Input: part model. Units: mm. Frame: model coordinates. A direction names the side the tool comes from. Coordinates: 2 decimals unless noted, no trailing zeros. Write each loop counter-clockwise with the first axis right and the second up, starting at its lowest first coordinate (ties: lowest second). Pieces come first, ordered by that corner, then holes. Notation, with made-up numbers: M 61,-16 L 99,-16 A32 cw 99,22 Z; hole C 65,27.25 d2. An arc over 180 degrees is marked long. Use CSV: the item, a comma, the result in double quotes.
```python
from build123d import *

# Parameters (mm, degrees)
SKETCH_1_W = 1.2
SKETCH_1_H = 5


with BuildPart() as part:
    # 草图1 → 旋转1 (revolve)
    with BuildSketch(Plane(origin=(0, 0, 0), x_dir=(1, 0, 0), z_dir=(0, 1, 0)), mode=Mode.PRIVATE) as revolve_1_sk:
        Polygon((0, 8.7), (0, 6), (1.45, 6), (2.95, 6), (2.95, 8.7), align=None)
        Polygon((0, 6), (0, 0), (1.2, 0), (1.45, 0), (1.45, 6), align=None)
        with Locations((0.6, -2.5)):
            Rectangle(SKETCH_1_W, SKETCH_1_H)
    revolve(revolve_1_sk.sketch.rotate(Axis((0, 0, -34.43030142), (0, 0, 1)), 180), axis=Axis((0, 0, -34.43030142), (0, 0, 1)))


solid = part.part
```
1. Section C-C (z = -5.75). Return loops of the section in (x, y).
Resolved:
outline,"C 0,0 d2.9"
2. Section D-D (y = 1.7). Return loops of the section in (x, z).
Resolved:
outline,"M -2.41,-8.7 L 2.41,-8.7 L 2.41,-6 L -2.41,-6 Z"
3. Section A-A (x = 0). Return loops of the section in (y, z).
Resolved:
outline,"M -2.95,-8.7 L 2.95,-8.7 L 2.95,-6 L 1.45,-6 L 1.45,0 L 1.2,0 L 1.2,5 L -1.2,5 L -1.2,0 L -1.45,0 L -1.45,-6 L -2.95,-6 Z"
4. Contact query for flat-ended pins moving along their axis: pin 1 Ø3 at (y, z) = (1, -2.5) entering from +X; pin 2 Ø3 at (x, z) = (-0.5, 2.5) entering from -Y; pin 3 Ø2 at (y, z) = (0, -4) entering from -X. Output: stop coordinate, or through.
Resolved:
pin 1,"stops at x = 1.45"
pin 2,"stops at y = -1.2"
pin 3,"stops at x = -1.45"
5. Material intervals for line 1 (Z direction, x = 0.5, y = 2.3); line 2 (Y direction, x = -2.3, z = -7); line 3 (Y direction, x = 1.3, z = -1.5), sorted ascending. Write a range as [from, to].
Resolved:
line 1,"z = [-8.7, -6]"
line 2,"y = [-1.85, 1.85]"
line 3,"y = [-0.64, 0.64]"
6. Access query for faces 1 (the flat face through (0, 0, -8.7)), 2 (the cylindrical face through (-1.38, -0.44, -3.04)). Directions: +Z, -Z, +X, -X, +Y, -Y. A direction counts if a zero-diameter tool reaches every point of the face in a straight line with its end or side. Return the directions, or none.
Resolved:
face 1,"-Z, +X, -X, +Y, -Y"
face 2,"+Z"
